Check sheet for the modelled part. Datum: model origin and axes. Units: mm. Face numbers are marked on the shaded views. A direction names the side the tool comes from. Give positions to 0.01 mm unless a question says otherwise; leave off trailing zeros. Order: outer loops, then holes, each group sorted by start corner. A loop starts at its lowest first (then second) coordinate and runs counter-clockwise, first axis right, second up.
```python
from build123d import *

# Parameters (mm, degrees)
SKETCH1_W           = 48
SKETCH1_H           = 8
SKETCH1_W_2         = 40.2
SKETCH1_H_2         = 4.2
BOSS_EXTRUDE1_DEPTH = 54
CUT_EXTRUDE1_START  = -3
SKETCH2_OUTSIDE_W   = 64.538
SKETCH2_OUTSIDE_H   = 24.538
CUT_EXTRUDE1_DEPTH  = 48
FILLET1_R           = 2
CHAMFER1_SIZE       = 1


with BuildPart() as part:
    # Sketch1 → Boss-Extrude1 (new body)
    with BuildSketch(Plane.XY):
        with Locations((24, 4)):
            Rectangle(SKETCH1_W, SKETCH1_H)
        with Locations((24, 4)):
            Rectangle(SKETCH1_W_2, SKETCH1_H_2, mode=Mode.SUBTRACT)
    extrude(amount=BOSS_EXTRUDE1_DEPTH)

    # Sketch2 outside → Cut-Extrude1 (cut)
    with BuildSketch(Plane.XY.offset(54).offset(CUT_EXTRUDE1_START)):
        with Locations((24, 4)):
            Rectangle(SKETCH2_OUTSIDE_W, SKETCH2_OUTSIDE_H)
        with BuildLine():
            Line((3.65, 6.85), (44.35, 6.85))
            ThreePointArc((44.35, 6.85), (44.703553391, 6.703553391), (44.85, 6.35))
            Line((44.85, 6.35), (44.85, 1.65))
            ThreePointArc((44.85, 1.65), (44.703553391, 1.296446609), (44.35, 1.15))
            Line((44.35, 1.15), (3.65, 1.15))
            ThreePointArc((3.65, 1.15), (3.296446609, 1.296446609), (3.15, 1.65))
            Line((3.15, 1.65), (3.15, 6.35))
            ThreePointArc((3.15, 6.35), (3.296446609, 6.703553391), (3.65, 6.85))
        make_face(mode=Mode.SUBTRACT)
    extrude(amount=-CUT_EXTRUDE1_DEPTH, mode=Mode.SUBTRACT)

    # Fillet1
    fillet1_edges = [part.edges().sort_by_distance(p)[0] for p in [
        (48, 0, 1.5),
        (0, 0, 1.5),
        (0, 8, 1.5),
        (48, 8, 1.5),
        (48, 0, 52.5),
        (0, 0, 52.5),
        (0, 8, 52.5),
        (48, 8, 52.5),
    ]]
    fillet(fillet1_edges, radius=FILLET1_R)

    # Chamfer1
    chamfer1_edges = [part.edges().sort_by_distance(p)[0] for p in [
        (3.15, 4, 3),
        (3.296446609, 1.296446609, 3),
        (24, 1.15, 3),
        (44.703553391, 1.296446609, 3),
        (44.85, 4, 3),
        (44.703553391, 6.703553391, 3),
        (24, 6.85, 3),
        (3.296446609, 6.703553391, 3),
        (3.296446609, 1.296446609, 51),
        (3.15, 4, 51),
        (3.296446609, 6.703553391, 51),
        (24, 6.85, 51),
        (44.703553391, 6.703553391, 51),
        (44.85, 4, 51),
        (44.703553391, 1.296446609, 51),
        (24, 1.15, 51),
    ]]
    chamfer(chamfer1_edges, length=CHAMFER1_SIZE)


solid = part.part
```
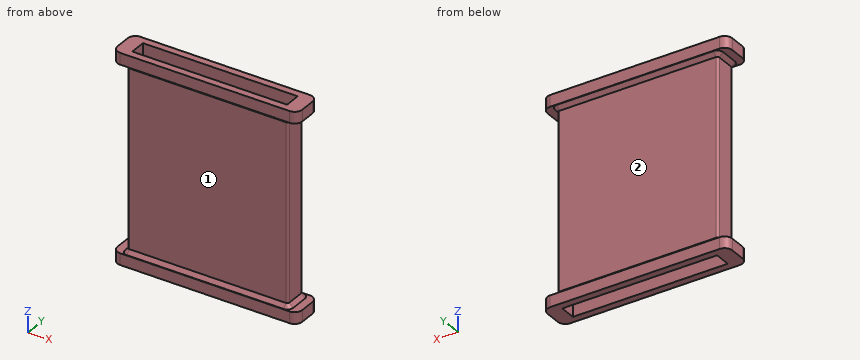
(1) Cross-section at C-C on z = 23.5. Enter the section's corners in (x, y).
Response values:
outline: (3.15, 1.65) arc R0.5 ccw to (3.65, 1.15) - (44.35, 1.15) arc R0.5 ccw to (44.85, 1.65) - (44.85, 6.35) arc R0.5 ccw to (44.35, 6.85) - (3.65, 6.85) arc R0.5 ccw to (3.15, 6.35) - close; hole (3.9, 1.9) - (44.1, 1.9) - (44.1, 6.1) - (3.9, 6.1) - close
(2) Gauge pin test, flat ends, axial feed: pin 1 Ø6 at (x, z) = (18.5, 33) entering from +Y; pin 2 Ø3.5 at (y, z) = (3.5, 17.5) entering from +X; pin 3 Ø2 at (x, z) = (23, 15.5) entering from -Y; pin 4 Ø2.5 at (x, y) = (32.5, 3) entering from -Z. Record the tip position at first contact, or that the pin passes through.
Response values:
pin 1: stops at y = 6.85
pin 2: stops at x = 44.85
pin 3: stops at y = 1.15
pin 4: stops at z = 0
(3) Material ranges on L1, parallel to Y at x = 44, z = 13; L2, parallel to X at y = 6, z = 22, recorded low to high.
Response values:
L1: y = 1.15 to 1.9, 6.1 to 6.85
L2: x = 3.15 to 3.9, 44.1 to 44.85
(4) Cross-section at A-A on x = 13.5. Enter the section's corners in (y, z), then the cut area to 3 significant figures.
Response values:
outline: (0, 0) - (1.9, 0) - (1.9, 54) - (0, 54) - (0, 51) - (0.15, 51) - (1.15, 50) - (1.15, 4) - (0.15, 3) - (0, 3) - close; (6.1, 0) - (8, 0) - (8, 3) - (7.85, 3) - (6.85, 4) - (6.85, 50) - (7.85, 51) - (8, 51) - (8, 54) - (6.1, 54) - close
area: 96.8 mm2
(5) Set-up check for the marked faces 1 and 2: record each of +Z, -Z, +X, -X, +Y, -Y from which the full face is reachable in a straight line by a thin tool's end or side.
Response values:
face 1: +X, -X, -Y
face 2: +X, -X, +Y
(6) Cross-section at B-B on y = 3.75. Enter the section's corners in (x, z).
Response values:
outline: (0, 0) - (3.9, 0) - (3.9, 54) - (0, 54) - (0, 51) - (2.15, 51) - (3.15, 50) - (3.15, 4) - (2.15, 3) - (0, 3) - close; (44.1, 0) - (48, 0) - (48, 3) - (45.85, 3) - (44.85, 4) - (44.85, 50) - (45.85, 51) - (48, 51) - (48, 54) - (44.1, 54) - close
